Print and shaded views of the part. All mm, measured from the part's lowest x, y and z. Coordinates: 2 decimals unless noted, no trailing zeros. Order: outer loops, then holes, each group sorted by start corner. A loop starts at its lowest first (then second) coordinate and runs counter-clockwise, first axis right, second up. Notation, with made-up numbers: (43, -3) - (96, -3) arc R19 ccw to (96, 11) - close; hole circle Ø2 at (17, 86.5). An arc over 180 degrees is marked (long way). Write each question's results on one line, items separated by ' | '.
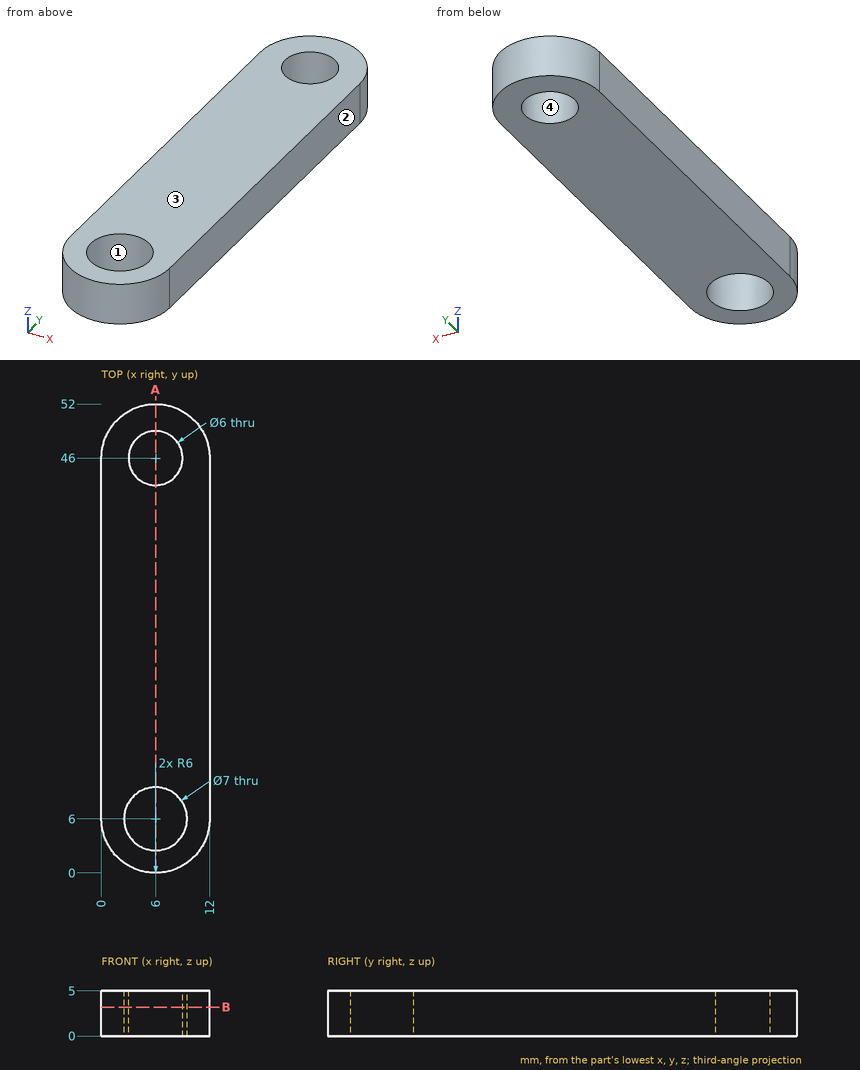
1. Band-saw the part on A-A on x = 6. Give the cut face in (y, z), then the cut area to 3 significant figures.
Solved:
outline: (0, 0) - (2.5, 0) - (2.5, 5) - (0, 5) - close; (9.5, 0) - (43, 0) - (43, 5) - (9.5, 5) - close; (49, 0) - (52, 0) - (52, 5) - (49, 5) - close | area: 195 mm2
2. Probe line 1 (Y direction, x = 6, z = 3.45); line 2 (Y direction, x = 8.5, z = 1.1); line 3 (X direction, y = 7.5, z = 2.9). List the from-to ranges inside material, lowest first.
Solved:
line 1: y = 0 to 2.5, 9.5 to 43, 49 to 52 | line 2: y = 0.55 to 3.55, 8.45 to 44.34, 47.66 to 51.45 | line 3: x = 0 to 2.84, 9.16 to 12
3. Two-plate mould, pull along X, no slides. Class the marked faces 1, 2, 3 and 4: +X half, -X half, draft (parallel to the pull), parting line (faces both ways), or undercut.
Solved:
face 1: undercut | face 2: +X half | face 3: draft | face 4: undercut
4. Band-saw the part on B-B on z = 3.2. Give the cut face in (x, y), then the cut area to 3 significant figures.
Solved:
outline: (0, 6) arc R6 ccw to (12, 6) - (12, 46) arc R6 ccw to (0, 46) - close; hole circle Ø7 at (6, 6); hole circle Ø6 at (6, 46) | area: 526 mm2
5. Drop flat-ended pins along their axis: pin 1 Ø4 at (x, y) = (6, 6) entering from +Z; pin 2 Ø2 at (x, z) = (8.5, 3.5) entering from -Y. Give the stop position or say it passes through.
Solved:
pin 1: passes through | pin 2: stops at y = 0.19
